from build123d import *

# Parameters (mm, degrees)
F0_W     = 228.6
F0_H     = 76.2
F1_DEPTH = 152.4
F2_W     = 152.4
F2_H     = 152.4
F2_H_2   = 76.2
F3_DEPTH = 76.2
F4_R     = 76.2
F5_R     = 76.19999


# Not quite as in the source:
# - a fillet or chamfer is up to 0.001 mm smaller than in the source, because OpenCascade refuses the exact size


with BuildPart() as f1:
    # F0 (on Front) → F1 (new body)
    with BuildSketch(Plane.XZ):
        with Locations((-3.7755966187, 13.4019921658)):
            Rectangle(F0_W, F0_H)
    extrude(amount=F1_DEPTH)

    # F2 (on face) → F3 (join)
    with BuildSketch(Plane.YZ.offset(110.5244033813)):
        with Locations((-76.2, 127.7019921658)):
            Rectangle(F2_W, F2_H)
        with Locations((-76.2, 13.4019921658)):
            Rectangle(F2_W, F2_H_2)
    extrude(amount=-F3_DEPTH)

    # F4
    f4_edges = [f1.edges().sort_by_distance(p)[0] for p in [
        (-3.775597, -152.4, -24.698008),
    ]]
    fillet(f4_edges, radius=F4_R)

    # F5 (radius 76.2 in the source; OpenCascade refuses exactly that, so slightly less here)
    f5_edges = [f1.edges().sort_by_distance(p)[0] for p in [
        (110.524403, -152.4, 127.701992),
    ]]
    fillet(f5_edges, radius=F5_R)


solid = f1.part
Part model, mm, in its own coordinate system. A direction names the side the tool comes from. Coordinates: 2 decimals unless noted, no trailing zeros. Order: outer loops, then holes, each group sorted by start corner. A loop starts at its lowest first (then second) coordinate and runs counter-clockwise, first axis right, second up. Notation, with made-up numbers: M 13.25,76 L 25.25,76 A28 cw 25.25,105 Z; hole C 82.25,71.25 d6. An arc over 180 degrees is marked long. Use a Markdown table: item, result.
(1) Cut at A-A on y = -35. Write the cut outline in (x, z).
A:
| item | result |
|---|---|
| outline | M -118.08,-24.7 L 34.32,-24.7 A76.2 ccw 110.52,51.5 L 110.52,203.9 L 34.32,203.9 L 34.32,51.5 L -118.08,51.5 Z |
(2) Probe L1, parallel to Y at x = 37, z = 107.5; L2, parallel to Z at x = -2.5, y = -38.5; L3, parallel to X at y = -77.5, z = 79.5. List the from-to ranges inside material, lowest first.
A:
| item | result |
|---|---|
| L1 | y = -152.35 to 0 |
| L2 | z = -24.7 to 51.5 |
| L3 | x = 34.32 to 110.51 |
(3) Tool access for faces 1 (the flat face through (-118.076, -75, 13)), 2 (the flat face through (34.324, -77, 129)): list every direction of +Z, -Z, +X, -X, +Y, -Y with a clear straight run to the whole face (end or side of a thin tool).
A:
| item | result |
|---|---|
| face 1 | +Z, -Z, -X, +Y, -Y |
| face 2 | +Z, -X, +Y, -Y |
(4) Cut at C-C on x = 2.5. Write the cut outline in (y, z).
A:
| item | result |
|---|---|
| outline | M -152.4,51.5 A76.2 ccw -76.2,-24.7 L 0,-24.7 L 0,51.5 Z |
(5) Flat gauge pins, fed straight in: pin 1 (5 mm diameter, centred on y = -47.5, z = 144.5, fed in from -X); pin 2 (3 mm diameter, centred on y = -83, z = 83, fed in from +X); pin 3 (1 mm diameter, centred on y = -67.5, z = -1, fed in from +X). Where does each tip first touch, or does it go through?
A:
| item | result |
|---|---|
| pin 1 | stops at x = 34.32 |
| pin 2 | stops at x = 110.34 |
| pin 3 | stops at x = 90.02 |
